Geometry check sheet. Reference: drawing and pictorial views, mm from the part's lowest x, y, z. A direction names the side the tool comes from. Coordinates: 2 decimals unless noted, no trailing zeros. Loops run counter-clockwise (first coordinate to the right, second up) from the corner with the lowest first, then second, coordinate; pieces in that order, holes last. Notation, with made-up numbers: (-12, 57.25) -> (46, 57.25) arc R17 cw to (46, 77.25) -> close; hole circle Ø4 at (43.25, 46.25). An arc over 180 degrees is marked (long way). Answer as a JSON object with one key per item and string values. Group by question number.
Q1. Set-up check for the marked faces 4, 5 and 6: record each of +Z, -Z, +X, -X, +Y, -Y from which the full face is reachable in a straight line by a thin tool's end or side.
Q2. Release check for a two-part mould opening along Y. For the marked faces 1, 2 and 3 record: released by +Y, released by -Y, zero draft, split by the parting line, or undercut.
Q3. Cross-section at C-C on x = 11.5. Record the boundary of the cut face in (y, z).
Q4. Scan lines: L1, parallel to Z at x = 69.5, y = 13.25; L2, parallel to X at y = 2, z = 11; L3, parallel to X at y = 6, z = 75.5. Record each from-to range of solid material in increasing order.
Q5. Cross-section at A-A on y = 4.75. Record the boundary of the cut face in (x, z) (1 decimal).
Q6. Gauge pin test, flat ends, axial feed: pin 1 Ø3 at (y, z) = (3, 57.5) entering from -X; pin 2 Ø15 at (x, y) = (6, 12) entering from -Z; pin 3 Ø3 at (y, z) = (5.5, 21.5) entering from -X. Record the tip position at first contact, or that the pin passes through.
Q7. Cross-section at B-B on z = 17. Record the boundary of the cut face in (x, y), and give its area (3 significant figures).
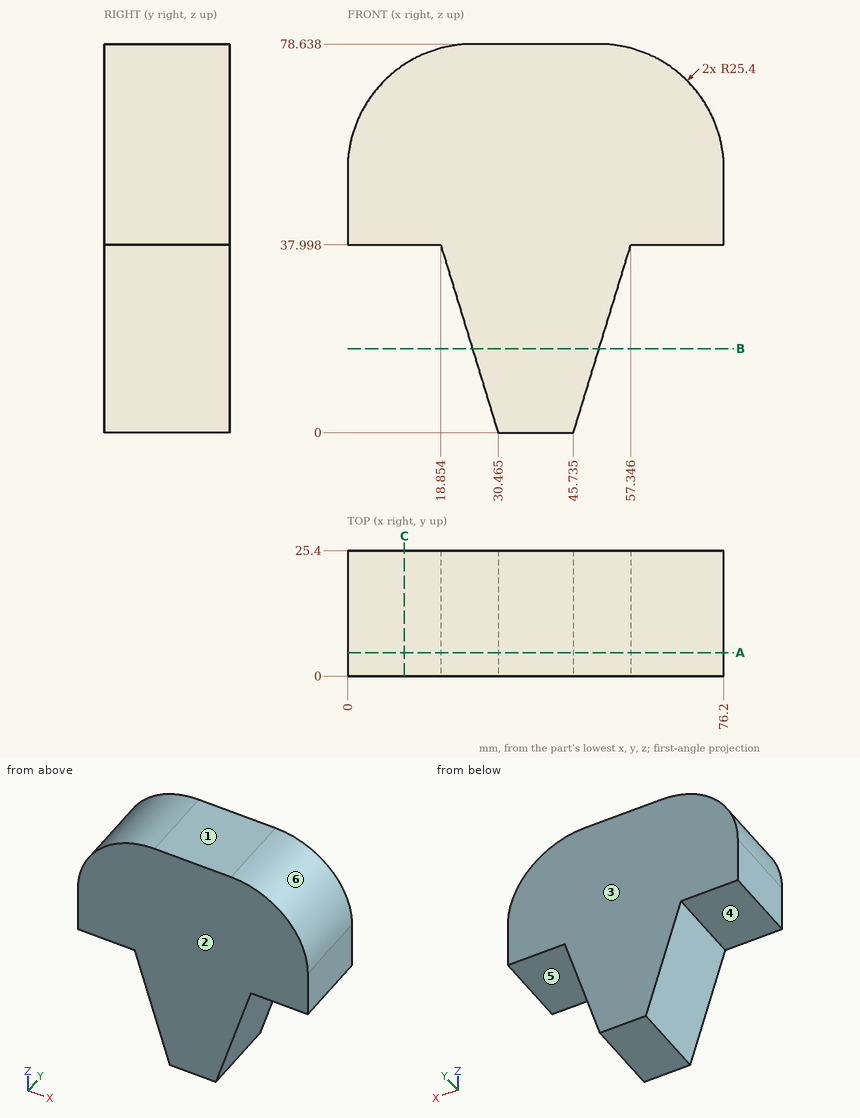
Computed values:
{
 "1": {"face 4": "-Z, -X, +Y, -Y", "face 5": "-Z, +X, +Y, -Y", "face 6": "+Z, +X, +Y, -Y"},
 "2": {"face 1": "zero draft", "face 2": "released by -Y", "face 3": "released by +Y"},
 "3": {"outline": "(0, 38) -> (25.4, 38) -> (25.4, 74.5) -> (0, 74.5) -> close"},
 "4": {"L1": "z = 38 to 70.43", "L2": "x = 27.1 to 49.1", "L3": "x = 13.17 to 63.03"},
 "5": {"outline": "(0, 38) -> (18.9, 38) -> (30.5, 0) -> (45.7, 0) -> (57.3, 38) -> (76.2, 38) -> (76.2, 53.2) arc R25.4 ccw to (50.8, 78.6) -> (25.4, 78.6) arc R25.4 ccw to (0, 53.2) -> close"},
 "6": {"pin 1": "stops at x = 0.15", "pin 2": "stops at z = 38", "pin 3": "stops at x = 23.44"},
 "7": {"outline": "(25.27, 0) -> (50.93, 0) -> (50.93, 25.4) -> (25.27, 25.4) -> close", "area": "652 mm²"}
}
